Geometry: see drawing. Coordinates: mm, zero at the bounding-box minimum. A direction names the side the tool comes from. Give positions to 0.01 mm unless a question says otherwise; leave off trailing zeros. Write each loop counter-clockwise with the first axis right and the second up, starting at its lowest first coordinate (ties: lowest second). Pieces come first, ordered by that corner, then holes. Notation, with made-up numbers: (57, 48.25) -> (89, 48.25) arc R13 ccw to (89, 67.25) -> close; hole circle Ø11 at (65, -1.5). An arc over 180 degrees is marked (long way). Write item = value, one per line.
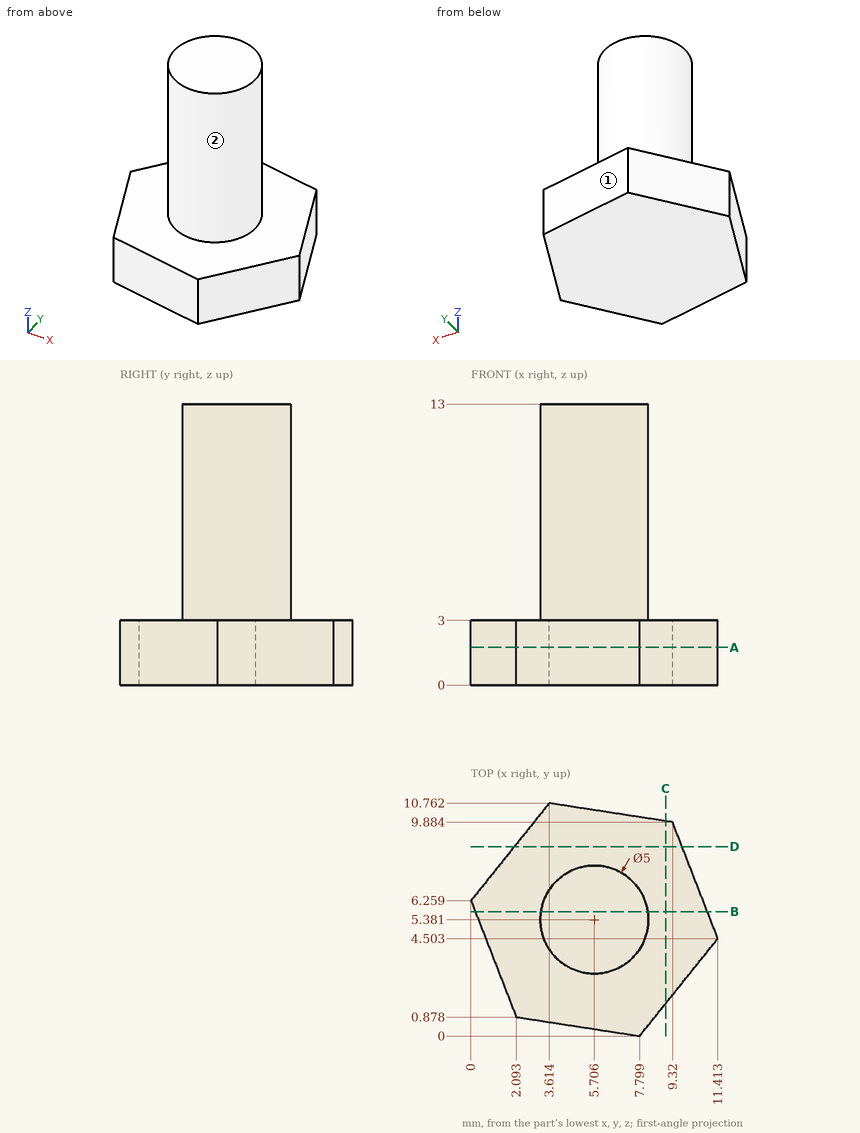
(1) First-contact query: pin 1 (3 mm diameter, centred on x = 8, y = 3, fed in from -Z); pin 2 (2 mm diameter, centred on y = 5.5, z = 8.5, fed in from -X). Flat tips, straight axial feed; report the tip coordinate or a pass-through.
Values follow:
pin_1 = 0
pin_2 = 3.21
(2) Section query A-A (z = 1.75). Return loops of the section in (x, y).
Values follow:
outline = (0, 6.26) -> (2.09, 0.88) -> (7.8, 0) -> (11.41, 4.5) -> (9.32, 9.88) -> (3.61, 10.76) -> close
(3) Section query D-D (y = 8.75). Return loops of the section in (x, z), plus the area to 3 significant figures.
Values follow:
outline = (2, 0) -> (9.76, 0) -> (9.76, 3) -> (2, 3) -> close
area = 23.3 mm2
(4) Section query B-B (y = 5.75). Return loops of the section in (x, z).
Values follow:
outline = (0.2, 0) -> (10.93, 0) -> (10.93, 3) -> (8.18, 3) -> (8.18, 13) -> (3.23, 13) -> (3.23, 3) -> (0.2, 3) -> close
(5) Material intervals for line 1 (Z direction, x = 6.75, y = 3); line 2 (X direction, y = 7, z = 2.5) (1 decimal); line 3 (X direction, y = 6.5, z = 4.5), sorted ascending.
Values follow:
line_1 = 0 to 3
line_2 = 0.6 to 10.4
line_3 = 3.47 to 7.94
(6) Access query for the marked faces 1 and 2. Directions: +Z, -Z, +X, -X, +Y, -Y. A direction counts if a zero-diameter tool reaches every point of the face in a straight line with its end or side. Return the directions, or none.
Values follow:
face_1 = +Z, -Z, +X, +Y
face_2 = +Z
(7) Section query C-C (x = 9). Return loops of the section in (y, z).
Values follow:
outline = (1.5, 0) -> (9.93, 0) -> (9.93, 3) -> (1.5, 3) -> close
